from build123d import *

# Parameters (mm, degrees)
SKETCH1_W                    = 180
SKETCH1_H                    = 15
BASE_FLANGE1_DEPTH           = 2.54
EDGE_FLANGE1_STRIP_W         = 11.6332
EDGE_FLANGE1_STRIP_H         = 2.54
EDGE_FLANGE1_STRIP_CUT_DEPTH = 180
EDGE_FLANGE1_DEPTH           = 180
EDGE_FLANGE2_STRIP_W         = 11.6332
EDGE_FLANGE2_STRIP_H         = 2.54
EDGE_FLANGE2_STRIP_CUT_DEPTH = 180
EDGE_FLANGE2_DEPTH           = 180
CUT_EXTRUDE3_DEPTH           = 92.167437169
CUT_EXTRUDE3_DEPTH_BACK      = 92.167437169
SKETCH12_R                   = 2.5
CUT_EXTRUDE4_DEPTH           = 92.167437169
CUT_EXTRUDE4_DEPTH_BACK      = 92.167437169
SKETCH16_R                   = 2
CUT_EXTRUDE6_DEPTH           = 92.549167118
FILLET1_R                    = 10
CUT_EXTRUDE7_DEPTH           = 93.088281556
CUT_EXTRUDE7_DEPTH_BACK      = 93.088281556
SKETCH18_R                   = 1.5


# Sheet-metal steps are written as plain solids
with BuildPart() as part:
    # Sketch1 → Base-Flange1 (new body)
    with BuildSketch(Plane(origin=(0, 0, 0), x_dir=(1, 0, 0), z_dir=(0, 1, 0))):
        Rectangle(SKETCH1_W, SKETCH1_H)
    extrude(amount=-BASE_FLANGE1_DEPTH)

    # Edge-Flange1 strip (across the edge) → Edge-Flange1 strip cut (cut)
    with BuildSketch(Plane(origin=(-90, 0, 7.5), x_dir=(0, 0, -1), z_dir=(1, 0, 0))):
        with Locations((-2.54, -1.27)):
            Rectangle(EDGE_FLANGE1_STRIP_W, EDGE_FLANGE1_STRIP_H)
    extrude(amount=EDGE_FLANGE1_STRIP_CUT_DEPTH, mode=Mode.SUBTRACT)

    # Edge-Flange1 section (across the edge) → Edge-Flange1 (add)
    with BuildSketch(Plane(origin=(-90, 0, 7.5), x_dir=(0, 0, -1), z_dir=(1, 0, 0))):
        with BuildLine():
            Line((0, 0.7366), (0, 12.46))
            Line((0, 12.46), (2.54, 12.46))
            Line((2.54, 12.46), (2.54, 0.7366))
            ThreePointArc((2.54, 0.7366), (2.755745145, 0.215745145), (3.2766, 0))
            Line((3.2766, 0), (3.2766, -2.54))
            ThreePointArc((3.2766, -2.54), (0.959693921, -1.580306079), (0, 0.7366))
        make_face()
    extrude(amount=EDGE_FLANGE1_DEPTH)

    # Edge-Flange2 strip (across the edge) → Edge-Flange2 strip cut (cut)
    with BuildSketch(Plane(origin=(90, 0, -7.5), x_dir=(0, 0, 1), z_dir=(-1, 0, 0))):
        with Locations((-2.54, -1.27)):
            Rectangle(EDGE_FLANGE2_STRIP_W, EDGE_FLANGE2_STRIP_H)
    extrude(amount=EDGE_FLANGE2_STRIP_CUT_DEPTH, mode=Mode.SUBTRACT)

    # Edge-Flange2 section (across the edge) → Edge-Flange2 (add)
    with BuildSketch(Plane(origin=(90, 0, -7.5), x_dir=(0, 0, 1), z_dir=(-1, 0, 0))):
        with BuildLine():
            Line((0, 0.7366), (0, 12.46))
            Line((0, 12.46), (2.54, 12.46))
            Line((2.54, 12.46), (2.54, 0.7366))
            ThreePointArc((2.54, 0.7366), (2.755745145, 0.215745145), (3.2766, 0))
            Line((3.2766, 0), (3.2766, -2.54))
            ThreePointArc((3.2766, -2.54), (0.959693921, -1.580306079), (0, 0.7366))
        make_face()
    extrude(amount=EDGE_FLANGE2_DEPTH)

    # Sketch12 → Cut-Extrude3 (cut, two sides: drawn at the far end of the back side and taken through both)
    with BuildSketch(Plane.XY.offset(-CUT_EXTRUDE3_DEPTH_BACK)):
        with Locations((75.835364308, 5.46)):
            Circle(SKETCH12_R)
    extrude(amount=CUT_EXTRUDE3_DEPTH + CUT_EXTRUDE3_DEPTH_BACK, mode=Mode.SUBTRACT)

    # Sketch16 → Cut-Extrude4 (cut, two sides: drawn at the far end of the back side and taken through both)
    with BuildSketch(Plane.XY.offset(-CUT_EXTRUDE4_DEPTH_BACK)):
        with Locations((-21.676425181, 4.934342186)):
            Circle(SKETCH16_R)
    extrude(amount=CUT_EXTRUDE4_DEPTH + CUT_EXTRUDE4_DEPTH_BACK, mode=Mode.SUBTRACT)

    # Sketch17 → Cut-Extrude6 (cut, through all)
    with BuildSketch(Plane.XZ.offset(2.54)):
        with BuildLine():
            Line((90, -3.5), (90, 3.5))
            Line((90, 3.5), (10, 3.5))
            ThreePointArc((10, 3.5), (12.474873734, 2.474873734), (13.5, 0))
            ThreePointArc((13.5, 0), (12.474873734, -2.474873734), (10, -3.5))
            Line((10, -3.5), (90, -3.5))
        make_face()
        with BuildLine():
            ThreePointArc((13.5, 0), (12.474873734, 2.474873734), (10, 3.5))
            Line((10, 3.5), (10, -3.5))
            ThreePointArc((10, -3.5), (12.474873734, -2.474873734), (13.5, 0))
        make_face()
        with BuildLine():
            Line((10, -3.5), (10, 3.5))
            ThreePointArc((10, 3.5), (6.5, 0), (10, -3.5))
        make_face()
    extrude(amount=-CUT_EXTRUDE6_DEPTH, mode=Mode.SUBTRACT)

    # Fillet1
    fillet1_edges = [part.edges().sort_by_distance(p)[0] for p in [
        (-90, 12.46, 6.23),
        (90, 12.46, 6.23),
        (90, 12.46, -6.23),
        (-90, 12.46, -6.23),
    ]]
    fillet(fillet1_edges, radius=FILLET1_R)

    # Sketch18 → Cut-Extrude7 (cut, two sides: drawn at the far end of the back side and taken through both)
    with BuildSketch(Plane(origin=(0, 0, -7.5), x_dir=(-1, 0, 0), z_dir=(0, 0, -1)).offset(-CUT_EXTRUDE7_DEPTH_BACK)):
        with Locations(Location((80, 6.7366, 0), (0, 0, 270))):
            Circle(SKETCH18_R)
    extrude(amount=CUT_EXTRUDE7_DEPTH + CUT_EXTRUDE7_DEPTH_BACK, mode=Mode.SUBTRACT)


solid = part.part
Geometry: final body of the model. Coordinates: model frame, mm. A direction names the side the tool comes from. Give positions to 0.01 mm unless a question says otherwise; leave off trailing zeros. Loops run counter-clockwise (first coordinate to the right, second up) from the corner with the lowest first, then second, coordinate; pieces in that order, holes last. Notation, with made-up numbers: (25, 1.25) - (44, 1.25) arc R16 cw to (44, 16.25) - close; hole circle Ø2 at (-5, -6.75). An arc over 180 degrees is marked (long way). One line per question, with ' | ' between items. Start each with the question number.
(1) Reachability of faces 4 (the cylindrical face through (-1.26, -1.61, 6.51)), 5 (the flat face through (-1, 7, 4.96)) from +Z, -Z, +X, -X, +Y, -Y: full face, straight path, thin tool, end or side. Return the list, or none.
(2) Section query B-B on x = -42. Return loops of the section in (y, z), then the cut area to 3 significant figures.
(3) Section query A-A on x = 65.5. Return loops of the section in (y, z).
(4) Section query C-C on z = 0.75. Return loops of the section in (x, y), then the cut area to 3 significant figures.
(5) Pull-direction query (Z, two-part tool) for faces 1 (the flat face through (-1, 7, 7.5)), 2 (the cylindrical face through (73.338, 5.57, -6.248)), 3 (the cylindrical face through (6.5, -1.3, 0.1)); classes: released by +Z, released by -Z, zero draft, split by the parting line, or undercut.
(6) Contact query for flat-ended pins moving along their axis: pin 1 (2 mm diameter, centred on x = 53.5, y = -1, fed in from -Z); pin 2 (2 mm diameter, centred on x = 55, y = -1, fed in from +Z). Output: stop coordinate, or through.
(7) Ray query, line 1 (Z direction, x = -61, y = 7.5); line 2 (X direction, y = 5.46, z = -6.9); line 3 (Y direction, x = -51, z = 3.75). Return the intervals inside material, ascending. Write a range as from..to.
The answers:
1) face 4: +Z, +X, -X, -Y | face 5: +X, -X, +Y
2) outline: (-2.54, -4.22) arc R3.28 ccw to (0.74, -7.5) - (12.46, -7.5) - (12.46, -4.96) - (0.74, -4.96) arc R0.74 cw to (0, -4.22) - (0, 4.22) arc R0.74 cw to (0.74, 4.96) - (12.46, 4.96) - (12.46, 7.5) - (0.74, 7.5) arc R3.28 ccw to (-2.54, 4.22) - close | area: 97.0 mm2
3) outline: (-2.54, -4.22) arc R3.28 ccw to (0.74, -7.5) - (12.46, -7.5) - (12.46, -4.96) - (0.74, -4.96) arc R0.74 cw to (0, -4.22) - (0, -3.5) - (-2.54, -3.5) - close; (-2.54, 3.5) - (0, 3.5) - (0, 4.22) arc R0.74 cw to (0.74, 4.96) - (12.46, 4.96) - (12.46, 7.5) - (0.74, 7.5) arc R3.28 ccw to (-2.54, 4.22) - close
4) outline: (-90, -2.54) - (6.58, -2.54) - (6.58, 0) - (-90, 0) - close | area: 245 mm2
5) face 1: released by +Z | face 2: zero draft | face 3: undercut
6) pin 1: z = -7.42 | pin 2: z = 7.42
7) line 1: -7.5..-4.96, 4.96..7.5 | line 2: -89.54..-80.79, -79.21..-23.61, -19.75..73.34, 78.34..89.54 | line 3: -2.54..0
